from build123d import *

# Parameters (mm, degrees)
F0_W     = 100
F0_H     = 60
F1_DEPTH = 60
F3_DEPTH = 100
F5_DEPTH = 73.8


with BuildPart() as f1:
    # F0 (on Front) → F1 (new body)
    with BuildSketch(Plane.XZ):
        with Locations((50, 30)):
            Rectangle(F0_W, F0_H)
    extrude(amount=F1_DEPTH)

    # F2 (on face) → F3 (cut)
    with BuildSketch(Plane(origin=(0, 0, 0), x_dir=(0, -1, 0), z_dir=(-1, 0, 0))):
        Polygon((0, 60), (60, 19.930851), (60, 60), align=None)
    extrude(amount=-F3_DEPTH, mode=Mode.SUBTRACT)

    # F4 (on face) → F5 (cut)
    with BuildSketch(Plane(origin=(0, 0, 0), x_dir=(1, 0, 0), z_dir=(0, 0, -1))):
        Polygon((100, 60), (69.933802, 60), (100, 15.354728), align=None)
    extrude(amount=-F5_DEPTH, mode=Mode.SUBTRACT)


solid = f1.part
The listing builds one solid part. Answer for the finished solid, in the listing's coordinates (mm). Round coordinates to 2 decimals unless told otherwise and drop trailing zeros. Order: outer loops, then holes, each group sorted by start corner. A loop starts at its lowest first (then second) coordinate and runs counter-clockwise, first axis right, second up. Notation, with made-up numbers: (85, 58.25) -> (118, 58.25) arc R23 ccw to (118, 88.25) -> close; hole circle Ø1 at (-30.5, 71.5). An arc over 180 degrees is marked (long way). Put each result on its own line as item: value.
Q1. Consider line 1 along X through (y, z) = (-22, 36); line 2 along Y through (x, z) = (7.5, 50); line 3 along Z through (x, y) = (13.5, -32.5). Determine where each line is inside the solid, lowest interval first.
Results list:
line 1: 0 to 95.52
line 2: -14.97 to 0
line 3: 0 to 38.3
Q2. Section B-B, the plane x = 62 is taken. Write down the section's boundary in (y, z).
Results list:
outline: (-60, 0) -> (0, 0) -> (0, 60) -> (-60, 19.93) -> close
Q3. Each of these flat-tipped pins is pushed along its axis until it touches: P1, Ø8, axis at x = 88.5, z = 10.5, coming from the -Y side; P2, Ø6, axis at x = 78, y = -48, coming from the +Z side; P3, Ø8, axis at x = 66, y = -9, coming from the +Z side. Where does it stop, or does it pass through?
Results list:
P1: y = -38.37
P2: z = 29.95
P3: z = 56.66
Q4. Section C-C, the plane y = -14 is taken. Write down the section's boundary in (x, z).
Results list:
outline: (0, 0) -> (100, 0) -> (100, 50.65) -> (0, 50.65) -> close
Q5. Section D-D, the plane z = 45.5 is taken. Write down the section's boundary in (x, y), and give its area (3 significant figures).
Results list:
outline: (0, -21.71) -> (95.72, -21.71) -> (100, -15.35) -> (100, 0) -> (0, 0) -> close
area: 2,160 mm^2
Q6. Section A-A, the plane z = 5 is taken. Write down the section's boundary in (x, y), and give its area (3 significant figures).
Results list:
outline: (0, -60) -> (69.93, -60) -> (100, -15.35) -> (100, 0) -> (0, 0) -> close
area: 5,330 mm^2
